Verification items for the finished model (mm, model axes). A direction names the side the tool comes from. Coordinates: 2 decimals unless noted, no trailing zeros. Answer in a Markdown table with one row per item.
```python
from build123d import *

# Parameters (mm, degrees)
SKIZZE1_W                       = 80
SKIZZE1_H                       = 195
AUFSATZ_LINEAR_AUSTRAGEN1_DEPTH = 10
SKIZZE2_R                       = 3.015
SKIZZE2_R_2                     = 15.25
SCHNITT_LINEAR_AUSTRAGEN1_DEPTH = 10
SKIZZE3_R                       = 1.25
SCHNITT_LINEAR_AUSTRAGEN2_DEPTH = 5
SKIZZE4_R                       = 2.5
SCHNITT_LINEAR_AUSTRAGEN3_DEPTH = 5
SKIZZE5_R                       = 1
SCHNITT_LINEAR_AUSTRAGEN4_DEPTH = 20
SCHNITT_LINEAR_START            = -30
SKIZZE6_R                       = 1
SCHNITT_LINEAR_AUSTRAGEN5_DEPTH = 30


with BuildPart() as part:
    # Skizze1 → Aufsatz-Linear austragen1 (new body)
    with BuildSketch(Plane.XY):
        with Locations((-29.059385344, -27.400468384)):
            Rectangle(SKIZZE1_W, SKIZZE1_H)
    extrude(amount=-AUFSATZ_LINEAR_AUSTRAGEN1_DEPTH)

    # Skizze2 → Schnitt-Linear austragen1 (cut)
    with BuildSketch(Plane(origin=(0, 0, -10), x_dir=(-1, 0, 0), z_dir=(0, 0, -1))):
        with Locations((18.659385344, 29.599531616)):
            Circle(SKIZZE2_R)
        with Locations((48.659385344, 29.599531616)):
            Circle(SKIZZE2_R)
        with Locations((18.659385344, -0.400468384)):
            Circle(SKIZZE2_R)
        with Locations((48.659385344, -0.400468384)):
            Circle(SKIZZE2_R)
        with Locations((33.659385344, 14.599531616)):
            Circle(SKIZZE2_R_2)
        with BuildLine():
            Line((23.241327633, -19.900468384), (23.241327633, -34.900468384))
            ThreePointArc((23.241327633, -34.900468384), (24.096006948, -36.96384678), (26.159385344, -37.818526095))
            Line((26.159385344, -37.818526095), (41.159385344, -37.818526095))
            ThreePointArc((41.159385344, -37.818526095), (43.22276374, -36.96384678), (44.077443055, -34.900468384))
            Line((44.077443055, -34.900468384), (44.077443055, -19.900468384))
            ThreePointArc((44.077443055, -19.900468384), (43.22276374, -17.837089988), (41.159385344, -16.982410673))
            Line((41.159385344, -16.982410673), (26.159385344, -16.982410673))
            ThreePointArc((26.159385344, -16.982410673), (24.096006948, -17.837089988), (23.241327633, -19.900468384))
        make_face()
    extrude(amount=-SCHNITT_LINEAR_AUSTRAGEN1_DEPTH, mode=Mode.SUBTRACT)

    # Skizze3 → Schnitt-Linear austragen2 (cut)
    with BuildSketch(Plane(origin=(0, 0, -10), x_dir=(-1, 0, 0), z_dir=(0, 0, -1))):
        with Locations((-5.940614656, 65.099531616)):
            Circle(SKIZZE3_R)
        with Locations((63.81594416, 65.099531616)):
            Circle(SKIZZE3_R)
        with Locations((28.937664752, 65.099531616)):
            Circle(SKIZZE3_R)
        with Locations((63.81594416, 42.599531616)):
            Circle(SKIZZE3_R)
        with Locations((63.81594416, -27.400468384)):
            Circle(SKIZZE3_R)
        with Locations((63.81594416, -97.400468384)):
            Circle(SKIZZE3_R)
        with Locations((63.81594416, -119.900468384)):
            Circle(SKIZZE3_R)
        with Locations((28.937664752, -119.900468384)):
            Circle(SKIZZE3_R)
        with Locations((-5.940614656, -119.900468384)):
            Circle(SKIZZE3_R)
        with Locations((-5.940614656, -97.400468384)):
            Circle(SKIZZE3_R)
        with Locations((-5.940614656, -27.400468384)):
            Circle(SKIZZE3_R)
        with Locations((-5.940614656, 42.599531616)):
            Circle(SKIZZE3_R)
    extrude(amount=-SCHNITT_LINEAR_AUSTRAGEN2_DEPTH, mode=Mode.SUBTRACT)

    # Skizze4 → Schnitt-Linear austragen3 (cut)
    with BuildSketch(Plane.XY):
        with Locations((-64.059385344, 65.099531616)):
            Circle(SKIZZE4_R)
        with Locations((5.940614656, 65.099531616)):
            Circle(SKIZZE4_R)
        with Locations((5.940614656, 42.599531616)):
            Circle(SKIZZE4_R)
        with Locations((5.940614656, -27.400468384)):
            Circle(SKIZZE4_R)
        with Locations((5.940614656, -97.400468384)):
            Circle(SKIZZE4_R)
        with Locations((5.940614656, -119.900468384)):
            Circle(SKIZZE4_R)
        with Locations((-64.059385344, -119.900468384)):
            Circle(SKIZZE4_R)
        with Locations((-64.059385344, -97.400468384)):
            Circle(SKIZZE4_R)
        with Locations((-64.059385344, -27.400468384)):
            Circle(SKIZZE4_R)
        with Locations((-64.059385344, 42.599531616)):
            Circle(SKIZZE4_R)
        with Locations((-29.059385344, -119.900468384)):
            Circle(SKIZZE4_R)
        with Locations((-29.059385344, 65.099531616)):
            Circle(SKIZZE4_R)
    extrude(amount=-SCHNITT_LINEAR_AUSTRAGEN3_DEPTH, mode=Mode.SUBTRACT)

    # Skizze5 → Schnitt-Linear austragen4 (cut)
    with BuildSketch(Plane.ZY.offset(69.059385344)):
        with Locations((-5, 29.599531616)):
            Circle(SKIZZE5_R)
        with Locations((-5, -0.400468384)):
            Circle(SKIZZE5_R)
    extrude(amount=-SCHNITT_LINEAR_AUSTRAGEN4_DEPTH, mode=Mode.SUBTRACT)

    # Skizze6 → Schnitt-Linear austragen5 (cut)
    with BuildSketch(Plane(origin=(10.940614656, 0, 0), x_dir=(0, 0, -1), z_dir=(1, 0, 0)).offset(SCHNITT_LINEAR_START)):
        with Locations(Location((5, 29.599531616, 0), (0, 0, 180))):
            Circle(SKIZZE6_R)
        with Locations(Location((5, -0.400468384, 0), (0, 0, 180))):
            Circle(SKIZZE6_R)
    extrude(amount=SCHNITT_LINEAR_AUSTRAGEN5_DEPTH, mode=Mode.SUBTRACT)


solid = part.part
```
1. Mould release check, pull along X, two halves, no side actions. Record for faces 3 (the flat face through (-21, -26, -10)), 4 (the flat face through (6, -96, -5)), 5 (the flat face through (-30, -121, -5)): released by +X, released by -X, zero draft, split by the parting line, or undercut.
Geometry says:
| item | result |
|---|---|
| face 3 | zero draft |
| face 4 | undercut |
| face 5 | undercut |
2. Section check A-A, the plane z = -2.25. State how many separate pieces and enclosed holes the cut face has, plus the area to 3 significant figures.
Geometry says:
| item | result |
|---|---|
| separate pieces | 1 |
| enclosed holes | 18 |
| area | 14,100 mm^2 |
3. Depth check by flat-ended pin: P1, Ø3, axis at x = 5.94, y = -27.4, coming from the +Z side; P2, Ø1.5, axis at x = -64, y = -119.5, coming from the +Z side; P3, Ø1.6, axis at y = 29.6, z = -5, coming from the +X side. Enter the tip coordinate at first touch or a pass-through.
Geometry says:
| item | result |
|---|---|
| P1 | z = -5 |
| P2 | through |
| P3 | x = -21.57 |
4. Thickness scan on line 1 (Y direction, x = -31, z = -7.25); line 2 (Y direction, x = -24, z = -1.25); line 3 (X direction, y = -33, z = -1). Record the ranges inside material, lowest first. Write a range as from..to.
Geometry says:
| item | result |
|---|---|
| line 1 | -124.9..-37.82, -16.98..-0.42, 29.62..70.1 |
| line 2 | -124.9..-36.86, -17.94..2.8, 26.4..70.1 |
| line 3 | -69.06..-44.08, -23.24..10.94 |
5. Tool access check on faces 1 (the flat face through (-34, -16.982, -5)), 2 (the cylindrical face through (5.4, -29.84, -2.46)). Record the directions out of +Z, -Z, +X, -X, +Y, -Y that give a thin tool (end or side, any length) a straight path to the whole face; none if there is none.
Geometry says:
| item | result |
|---|---|
| face 1 | +Z, -Z |
| face 2 | +Z |
